from build123d import *

# Parameters (mm, degrees)
CROQUIS1_R                 = 75
CROQUIS1_R_2               = 61.225
SALIENTE_EXTRUIR1_DEPTH    = 15
CORTAR_EXTRUIR3_START      = 15
CROQUIS1_4_OUTSIDE_W       = 194.532
CROQUIS1_4_OUTSIDE_H       = 194.532
CROQUIS1_4_OUTSIDE_R       = 75
CROQUIS1_4_OUTSIDE_R_2     = 61.225
CORTAR_EXTRUIR3_DEPTH      = 1.5
CORTAR_EXTRUIR5_DEPTH      = 107.921700323
CORTAR_EXTRUIR5_DEPTH_BACK = 107.921700323
CROQUIS2_R                 = 2.5
CORTAR_EXTRUIR6_DEPTH      = 5.2
CORTAR_EXTRUIR6_DEPTH_BACK = 107.921700323
CORTAR_EXTRUIR6_START      = -13.5
CROQUIS2_4_R               = 4.25
CROQUIS3_R                 = 2.5
CORTAR_EXTRUIR7_DEPTH      = 10


with BuildPart() as part:
    # Croquis1 → Saliente-Extruir1 (new body)
    # profile 1 of 2: a face of its own
    with BuildSketch(Plane(origin=(0, 0, 0), x_dir=(1, 0, 0), z_dir=(0, 1, 0))):
        with Locations(Location((0, 0, 0), (0, 0, 270))):
            Circle(CROQUIS1_R)
        Circle(CROQUIS1_R_2, mode=Mode.SUBTRACT)
    # profile 2 of 2: a face of its own
    with BuildSketch(Plane(origin=(0, 0, 0), x_dir=(1, 0, 0), z_dir=(0, 1, 0))):
        Circle(CROQUIS1_R_2)
    extrude(amount=SALIENTE_EXTRUIR1_DEPTH)

    # Croquis1<4> outside → Cortar-Extruir3 (cut)
    # profile 1 of 2: a face of its own
    with BuildSketch(Plane(origin=(0, 0, 0), x_dir=(1, 0, 0), z_dir=(0, 1, 0)).offset(CORTAR_EXTRUIR3_START)):
        Rectangle(CROQUIS1_4_OUTSIDE_W, CROQUIS1_4_OUTSIDE_H)
        with Locations(Location((0, 0, 0), (0, 0, 270))):
            Circle(CROQUIS1_4_OUTSIDE_R, mode=Mode.SUBTRACT)
    # profile 2 of 2: a face of its own
    with BuildSketch(Plane(origin=(0, 0, 0), x_dir=(1, 0, 0), z_dir=(0, 1, 0)).offset(CORTAR_EXTRUIR3_START)):
        with Locations(Location((0, 0, 0), (0, 0, 270))):
            Circle(CROQUIS1_4_OUTSIDE_R_2)
    extrude(amount=-CORTAR_EXTRUIR3_DEPTH, mode=Mode.SUBTRACT)

    # Croquis2 → Cortar-Extruir5 (cut, two sides: drawn at the far end of the back side and taken through both)
    with BuildSketch(Plane(origin=(0, 13.5, 0), x_dir=(1, 0, 0), z_dir=(0, 1, 0)).offset(-CORTAR_EXTRUIR5_DEPTH_BACK)):
        with Locations(Location((-35.338232438, 14.241465098, 0), (0, 0, 270))):
            Circle(CROQUIS2_R)
        with Locations(Location((-5.335645657, 37.724539565, 0), (0, 0, 270))):
            Circle(CROQUIS2_R)
        with Locations(Location((30.002586781, 23.483074467, 0), (0, 0, 270))):
            Circle(CROQUIS2_R)
        with Locations(Location((35.338232438, -14.241465098, 0), (0, 0, 270))):
            Circle(CROQUIS2_R)
        with Locations(Location((5.335645657, -37.724539565, 0), (0, 0, 270))):
            Circle(CROQUIS2_R)
        with Locations(Location((-30.002586781, -23.483074467, 0), (0, 0, 270))):
            Circle(CROQUIS2_R)
    extrude(amount=CORTAR_EXTRUIR5_DEPTH + CORTAR_EXTRUIR5_DEPTH_BACK, mode=Mode.SUBTRACT)

    # Croquis2<4> → Cortar-Extruir6 (cut, two sides: drawn at the far end of the back side and taken through both)
    with BuildSketch(Plane(origin=(0, 13.5, 0), x_dir=(1, 0, 0), z_dir=(0, 1, 0)).offset(CORTAR_EXTRUIR6_START - CORTAR_EXTRUIR6_DEPTH_BACK)):
        with Locations(Location((-35.338232438, 14.241465098, 0), (0, 0, 270))):
            Circle(CROQUIS2_4_R)
        with Locations((-4.027016235, 36.022318165)):
            Circle(CROQUIS2_4_R)
        with Locations((30.491363939, 19.796436043)):
            Circle(CROQUIS2_4_R)
        with Locations((33.698527909, -18.210299146)):
            Circle(CROQUIS2_4_R)
        with Locations((2.387311706, -39.991152213)):
            Circle(CROQUIS2_4_R)
        with Locations((-32.131068468, -23.765270091)):
            Circle(CROQUIS2_4_R)
    extrude(amount=CORTAR_EXTRUIR6_DEPTH + CORTAR_EXTRUIR6_DEPTH_BACK, mode=Mode.SUBTRACT)

    # Croquis3 → Cortar-Extruir7 (cut)
    with BuildSketch(Plane.XZ):
        with Locations(Location((35.040630993, 53.555151962, 0), (0, 0, 270))):
            Circle(CROQUIS3_R)
        with Locations(Location((-53.555151962, 35.040630993, 0), (0, 0, 270))):
            Circle(CROQUIS3_R)
        with Locations(Location((53.555151962, -35.040630993, 0), (0, 0, 270))):
            Circle(CROQUIS3_R)
        with Locations(Location((-35.040630993, -53.555151962, 0), (0, 0, 270))):
            Circle(CROQUIS3_R)
    extrude(amount=-CORTAR_EXTRUIR7_DEPTH, mode=Mode.SUBTRACT)


solid = part.part
Design review of the part built by this model. Coordinates are the model's own, in mm. A direction names the side the tool comes from. Coordinates: 2 decimals unless noted, no trailing zeros. Order: outer loops, then holes, each group sorted by start corner. A loop starts at its lowest first (then second) coordinate and runs counter-clockwise, first axis right, second up. Notation, with made-up numbers: (50, -7.5) - (74, -7.5) arc R22 ccw to (74, 11.5) - close; hole circle Ø7 at (65.25, 38). An arc over 180 degrees is marked (long way). Put each result on its own line as item: value.
1) Insertion check: P1, Ø6, axis at x = -35.04, z = -53.56, coming from the -Y side; P2, Ø3, axis at y = 11.5, z = -24, coming from the +X side; P3, Ø4, axis at x = -32, z = 23.5, coming from the -Y side; P4, Ø5, axis at y = 11.5, z = -15, coming from the +X side. Each pin has a flat end and moves straight along its axis. Give the tip position at first contact, or say it passes through.
Response values:
P1: stops at y = 0
P2: stops at x = 71.55
P3: stops at y = 5.2
P4: stops at x = 73.95
2) Tool access review of faces 3 (the face through (35.448, 6.656, 11.744)), 4 (the face through (32.823, 4.93, 52.402)), 5 (the face through (-37.25, 14.26, -48.59)): name each direction out of +Z, -Z, +X, -X, +Y, -Y from which nothing blocks a thin tool from reaching the whole face with its end or side.
Response values:
face 3: +Y, -Y
face 4: -Y
face 5: +Y
3) Take a section at B-B, the plane x = -49. Give the boundary of the cut face in (y, z).
Response values:
outline: (0, -56.78) - (15, -56.78) - (15, -36.71) - (13.5, -36.71) - (13.5, 36.71) - (15, 36.71) - (15, 56.78) - (0, 56.78) - close
4) The part is to be moulded in two halves that separate along Z. For faces 1 (the face through (54, 10, -35)), 2 (the face through (-1, 0, -1)), say which applies: released by +Z, released by -Z, zero draft, split by the parting line, or undercut.
Response values:
face 1: undercut
face 2: zero draft
5) Wall thickness on L1, parallel to Z at x = 2, y = 2; L2, parallel to Y at x = 25, z = 30; L3, parallel to X at y = 7, z = -13.5 (3 decimals): over which ranges is each line inside the solid? List them lowest first. Write a range as from..to.
Response values:
L1: z = -74.97..35.76, 44.22..74.97
L2: y = 0..13.5
L3: x = -73.775..-37.726, -32.951..73.775
6) Take a section at A-A, the plane z = 0. Give the boundary of the cut face in (x, y) (3 decimals).
Response values:
outline: (-75, 0) - (75, 0) - (75, 15) - (61.225, 15) - (61.225, 13.5) - (-61.225, 13.5) - (-61.225, 15) - (-75, 15) - close
